from build123d import *

# Parameters (mm, degrees)
SKETCH1_R           = 4.7625
BOSS_EXTRUDE1_DEPTH = 9.525
SKETCH2_R           = 3.175
BOSS_EXTRUDE2_DEPTH = 6.35
SKETCH3_R           = 2.0574
BOSS_EXTRUDE3_DEPTH = 3.81
SKETCH4_W           = 0.79375
SKETCH4_H           = 3.175
BOSS_EXTRUDE4_DEPTH = 5.842
FILLET1_R           = 0.254


with BuildPart() as part:
    # Sketch1 → Boss-Extrude1 (new body)
    with BuildSketch(Plane(origin=(0, 0, 0), x_dir=(1, 0, 0), z_dir=(0, 1, 0))):
        Circle(SKETCH1_R)
    extrude(amount=-BOSS_EXTRUDE1_DEPTH)

    # Sketch2 → Boss-Extrude2 (add)
    with BuildSketch(Plane(origin=(0, 0, 0), x_dir=(1, 0, 0), z_dir=(0, 1, 0))):
        Circle(SKETCH2_R)
    extrude(amount=BOSS_EXTRUDE2_DEPTH)

    # Sketch3 → Boss-Extrude3 (add)
    with BuildSketch(Plane(origin=(0, 6.35, 0), x_dir=(1, 0, 0), z_dir=(0, 1, 0))):
        Circle(SKETCH3_R)
    extrude(amount=BOSS_EXTRUDE3_DEPTH)

    # Sketch4 → Boss-Extrude4 (add)
    with BuildSketch(Plane.XZ.offset(9.525)):
        with Locations((2.921, 0)):
            Rectangle(SKETCH4_W, SKETCH4_H)
        with Locations((-2.921, 0)):
            Rectangle(SKETCH4_W, SKETCH4_H)
    extrude(amount=BOSS_EXTRUDE4_DEPTH)

    # Fillet1
    fillet1_edges = [part.edges().sort_by_distance(p)[0] for p in [
        (-2.0574, 10.16, 0),
    ]]
    fillet(fillet1_edges, radius=FILLET1_R)


solid = part.part
Source: CAD feature listing. Evaluate the final solid. Frame: model axes, mm. A direction names the side the tool comes from. Give positions to 0.01 mm unless a question says otherwise; leave off trailing zeros. Loops run counter-clockwise (first coordinate to the right, second up) from the corner with the lowest first, then second, coordinate; pieces in that order, holes last. Notation, with made-up numbers: (75.5, 58) -> (115.5, 58) arc R37 ccw to (115.5, 95) -> close; hole circle Ø2 at (45, -35.75). An arc over 180 degrees is marked (long way). Use a Markdown table: item, result. Add a question column.
1) Section query A-A, the plane y = -13.5. Return the cut outline in (x, z), then the cut area to 3 significant figures.
2) Pull-direction query (X, two-part tool) for faces 1 (the face through (0, -9.525, 0)), 2 (the face through (-3.78, -4.7, 2.9)), 3 (the face through (3.318, -12, 0)), 4 (the face through (2.524, -12, 0)); classes: +X half, -X half, draft (parallel to the pull), parting line (faces both ways), or undercut.
3) Reachability of faces 5 (the face through (-2.524, -12, 0)), 6 (the face through (-3.318, -12, 0)), 7 (the face through (-2.055, 8.103, -0.09)) from +Z, -Z, +X, -X, +Y, -Y: full face, straight path, thin tool, end or side. Return the list, or none.
4) Section query D-D, the plane y = -3.25. Return the cut outline in (x, z) (1 decimal), then the cut area to 3 significant figures.
5) First-contact query: pin 1 (2.5 mm diameter, centred on y = -13.5, z = -0.5, fed in from -X); pin 2 (2 mm diameter, centred on x = 1, y = -7.5, fed in from -Z); pin 3 (2 mm diameter, centred on x = -2, y = -5, fed in from +Z); pin 4 (2.5 mm diameter, centred on y = -11.5, z = -0.5, fed in from +X). Flat tips, straight axial feed; report the tip coordinate or a pass-through.
6) Line query: line 1 along X through (y, z) = (-14.5, 1.25); line 2 along Y through (x, z) = (-0.75, -4) (3 decimals); line 3 along Y through (x, z) = (0.25, -2.25) (3 decimals). Output: solid intervals per line, ascending. Write a range as [from, to].
Numbers:
| question | item | result |
|---|---|---|
| 1 | outline | (-3.32, -1.59) -> (-2.52, -1.59) -> (-2.52, 1.59) -> (-3.32, 1.59) -> close; (2.52, -1.59) -> (3.32, -1.59) -> (3.32, 1.59) -> (2.52, 1.59) -> close |
| 1 | area | 5.04 mm2 |
| 2 | face 1 | undercut |
| 2 | face 2 | parting line |
| 2 | face 3 | +X half |
| 2 | face 4 | undercut |
| 3 | face 5 | +Z, -Z, -Y |
| 3 | face 6 | +Z, -Z, -X, -Y |
| 3 | face 7 | +Y |
| 4 | outline | circle Ø9.5 at (0, 0) |
| 4 | area | 71.3 mm2 |
| 5 | pin 1 | stops at x = -3.32 |
| 5 | pin 2 | stops at z = -4.76 |
| 5 | pin 3 | stops at z = 4.66 |
| 5 | pin 4 | stops at x = 3.32 |
| 6 | line 1 | x = [-3.32, -2.52], [2.52, 3.32] |
| 6 | line 2 | y = [-9.525, 0] |
| 6 | line 3 | y = [-9.525, 6.35] |
